Work out the finished part from the listing and answer in its coordinate system (mm). A direction names the side the tool comes from. Give positions to 0.01 mm unless a question says otherwise; leave off trailing zeros. Order: outer loops, then holes, each group sorted by start corner. A loop starts at its lowest first (then second) coordinate and runs counter-clockwise, first axis right, second up. Notation, with made-up numbers: M 53,65 L 89,65 A21 cw 89,73 Z; hole C 49,-28.5 d2. An arc over 180 degrees is marked long. One line per item, written item: value.
from build123d import *

# Parameters (mm, degrees)
SKETCH_1_W      = 35
SKETCH_1_H      = 35
EXTRUDE_1_DEPTH = 39
SKETCH_2_R      = 11
EXTRUDE_2_DEPTH = 2
EXTRUDE_3_DEPTH = 17
CHAMFER_1_SIZE  = 3


with BuildPart() as part:
    # 草图1 → 凸台-拉伸1 (new body)
    with BuildSketch(Plane.XY):
        Rectangle(SKETCH_1_W, SKETCH_1_H)
    extrude(amount=EXTRUDE_1_DEPTH)

    # 草图2 → 凸台-拉伸2 (add)
    with BuildSketch(Plane(origin=(0, 0, 0), x_dir=(-1, 0, 0), z_dir=(0, 0, -1))):
        Circle(SKETCH_2_R)
    extrude(amount=EXTRUDE_2_DEPTH)

    # 草图3 → 凸台-拉伸3 (add)
    with BuildSketch(Plane(origin=(0, 0, -2), x_dir=(-1, 0, 0), z_dir=(0, 0, -1))):
        with BuildLine():
            Line((-1.5, 2), (1.5, 2))
            ThreePointArc((1.5, 2), (0, -2.5), (-1.5, 2))
        make_face()
    extrude(amount=EXTRUDE_3_DEPTH)

    # 倒角1
    chamfer_1_edges = [part.edges().sort_by_distance(p)[0] for p in [
        (17.5, -17.5, 19.5),
        (-17.5, -17.5, 19.5),
        (-17.5, 17.5, 19.5),
        (17.5, 17.5, 19.5),
    ]]
    chamfer(chamfer_1_edges, length=CHAMFER_1_SIZE)


solid = part.part
(1) Section A-A, the plane x = 0 is taken. Give the vertices of the cut face in (y, z).
Findings:
outline: M -17.5,0 L -11,0 L -11,-2 L -2.5,-2 L -2.5,-19 L 2,-19 L 2,-2 L 11,-2 L 11,0 L 17.5,0 L 17.5,39 L -17.5,39 Z
(2) Section B-B, the plane y = 0 is taken. Give the vertices of the cut face in (x, z), then the cut area to 3 significant figures.
Findings:
outline: M -17.5,0 L -11,0 L -11,-2 L -2.5,-2 L -2.5,-19 L 2.5,-19 L 2.5,-2 L 11,-2 L 11,0 L 17.5,0 L 17.5,39 L -17.5,39 Z
area: 1,490 mm^2
(3) Given P1, Ø1, axis at x = 8, z = -1, coming from the -Y side; P2, Ø3, axis at y = -2.5, z = -12, coming from the +X side; P3, Ø12, axis at x = -3.5, y = -9, coming from the -Z side, each flat-ended and moving along its own axis, determine where each tip first touches the part or whether it passes through.
Findings:
P1: stops at y = -8.05
P2: stops at x = 2.29
P3: stops at z = -2
(4) Find the intervals of material crossed by probe 1 along Z at (x, y) = (-15.5, 3.5); probe 2 along Z at (x, y) = (8, -4); probe 3 along X at (y, z) = (1, -15.5), in increasing order. Write a range as from..to.
Findings:
probe 1: z = 0..39
probe 2: z = -2..39
probe 3: x = -2.29..2.29
(5) Which of the six approach directions +Z, -Z, +X, -X, +Y, -Y give full straight-line access (tool end or side, diameter ignored) to faces 1 (the cylindrical face through (-0.1, -2.5, -10.4)), 2 (the flat face through (0, 17.5, 19)), 3 (the flat face through (0, 2, -10))?
Findings:
face 1: -Z
face 2: +Z, -Z, +X, -X, +Y
face 3: -Z, +X, -X, +Y
(6) Section C-C, the plane z = -1 is taken. Give the vertices of the cut face in (x, y), then the cut area to 3 significant figures.
Findings:
outline: C 0,0 d22
area: 380 mm^2
(7) Section D-D, the plane x = 10 is taken. Give the vertices of the cut face in (y, z), then the cut area to 3 significant figures.
Findings:
outline: M -17.5,0 L -4.58,0 L -4.58,-2 L 4.58,-2 L 4.58,0 L 17.5,0 L 17.5,39 L -17.5,39 Z
area: 1,380 mm^2
